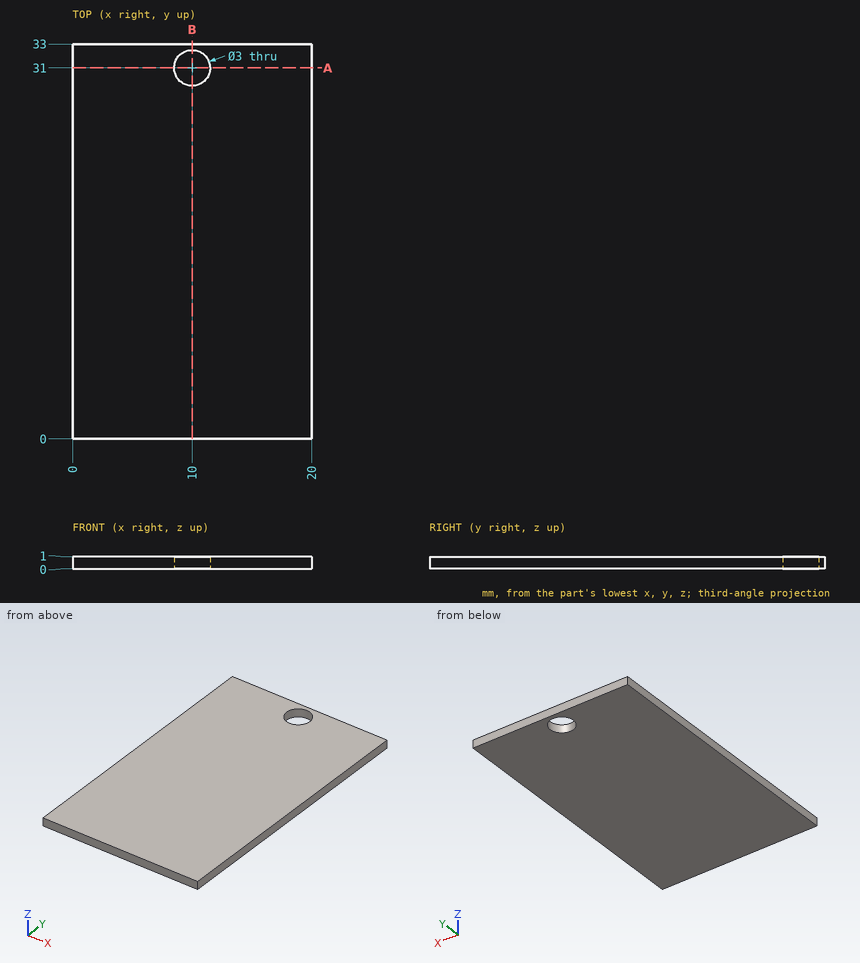
Verification items for this drawing (mm, ordinates from the low corner). Give positions to 0.01 mm unless a question says otherwise; leave off trailing zeros. Write each loop counter-clockwise with the first axis right and the second up, starting at its lowest first coordinate (ties: lowest second). Pieces come first, ordered by that corner, then holes.
1) Cross-section at A-A (y = 31). Record the boundary of the cut face in (x, z).
Values follow:
outline: (0, 0) - (8.5, 0) - (8.5, 1) - (0, 1) - close; (11.5, 0) - (20, 0) - (20, 1) - (11.5, 1) - close
2) Thickness scan on line 1 (X direction, y = 31, z = 0.35); line 2 (Y direction, x = 10, z = 0.6); line 3 (X direction, y = 30, z = 0.25). Record the ranges inside material, lowest first.
Values follow:
line 1: x = 0 to 8.5, 11.5 to 20
line 2: y = 0 to 29.5, 32.5 to 33
line 3: x = 0 to 8.88, 11.12 to 20
3) Cross-section at B-B (x = 10). Record the boundary of the cut face in (y, z), plus the area to 3 significant figures.
Values follow:
outline: (0, 0) - (29.5, 0) - (29.5, 1) - (0, 1) - close; (32.5, 0) - (33, 0) - (33, 1) - (32.5, 1) - close
area: 30.0 mm2
